Model file for the job. Use its own axes, mm. Face numbers are marked on the shaded views. A direction names the side the tool comes from. Give positions to 0.01 mm unless a question says otherwise; leave off trailing zeros. Write each loop counter-clockwise with the first axis right and the second up, starting at its lowest first coordinate (ties: lowest second). Pieces come first, ordered by that corner, then holes. Notation, with made-up numbers: (-25, -33) - (-17, -33) arc R26 ccw to (-17, 6) - close; hole circle Ø5 at (70, 41.5). An arc over 180 degrees is marked (long way). One line per item, written item: value. Start each with the question number.
(1) Drop flat-ended pins along their axis: P1, Ø2, axis at y = -4.5, z = -26.5, coming from the -X side; P2, Ø9, axis at x = 89, z = -82, coming from the +Y side; P3, Ø1.5, axis at y = -8, z = -61, coming from the +X side; P4, Ø1.5, axis at x = 46.5, z = -10.5, coming from the -Y side. Give the stop position or say it passes through.
(2) 3-axis set-ups, long thin cutter, end or side, ignore diameter. For the marked faces 1, 2 and 3: which of +Z, -Z, +X, -X, +Y, -Y reach the whole face in a straight line?
(3) Cut at B-B, the plane y = -10. List the corners of the cut face in (x, z) (3 decimals), and give its area (3 significant figures).
(4) Cut at A-A, the plane x = 32. List the corners of the cut face in (y, z) (3 decimals), and give its area (3 significant figures).
(5) Probe L1, parallel to Z at x = 35, y = 0.25; L2, parallel to X at y = -11.5, z = -58; L3, parallel to Y at x = 60.5, z = -10.5. List the from-to ranges inside material, lowest first.
(6) Cut at D-D, the plane x = 10. List the corners of the cut face in (y, z) (3 decimals).
(7) Cut at C-C, the plane z = -14.5. List the corners of the cut face in (x, y), and give its area (3 significant figures).
(8) Mould opens along X. For the marked faces 4, 5 and 6 say: pulls with the +X half, pulls with the -X half, needs draft (parallel to the pull), parting line crosses it, or undercut.
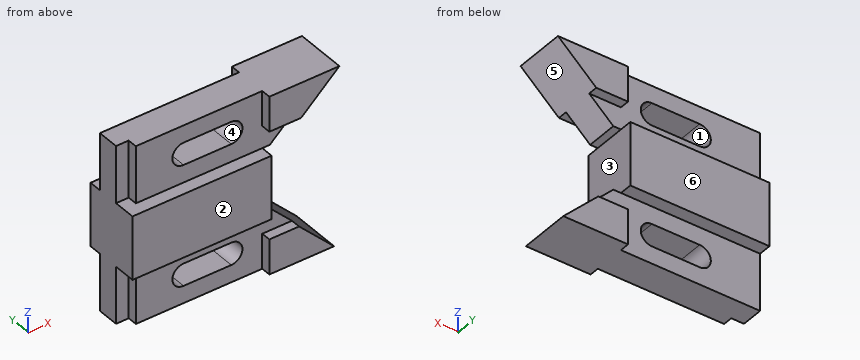
from build123d import *

# Parameters (mm, degrees)
F1_DEPTH = 14.224
F2_DEPTH = 7.874
F3_DEPTH = 12.7
F0_W     = 6.35
F0_H     = 28.575
F4_DEPTH = 7.874
F5_W     = 6.35
F5_H     = 28.575
F6_DEPTH = 4.826
F8_DEPTH = 22.099


with BuildPart() as f1:
    # F0 (on Front) → F1 (new body, symmetric)
    with BuildSketch(Plane.XZ):
        Polygon((6.35, -28.575), (0, -28.575), (0, -44.45), (0, -60.325), (6.35, -60.325), (69.596, -60.325), (69.596, -28.575), align=None)
    extrude(amount=F1_DEPTH, both=True)

    # F0 (on Front) → F2 (join, symmetric)
    with BuildSketch(Plane.XZ):
        Polygon((69.596, -60.325), (6.35, -60.325), (6.35, -88.9), (69.596, -88.9), (69.596, -71.374), (84.455, -71.374), (73.406, -60.325), align=None)
        Polygon((69.596, 0), (6.35, 0), (6.35, -28.575), (69.596, -28.575), (73.406, -28.575), (85.48624, -17.526), (69.596, -17.526), align=None)
    extrude(amount=F2_DEPTH, both=True)

    # F0 (on Front) → F3 (join, symmetric)
    with BuildSketch(Plane.XZ):
        Polygon((104.648, 0), (69.596, 0), (69.596, -17.526), (85.48624, -17.526), align=None)
        Polygon((69.596, -71.374), (69.596, -88.9), (101.981, -88.9), (84.455, -71.374), align=None)
    extrude(amount=F3_DEPTH, both=True)

    # F0 (on Front) → F4 (join, symmetric)
    with BuildSketch(Plane.XZ):
        with Locations((3.175, -14.2875)):
            Rectangle(F0_W, F0_H)
        Polygon((6.35, -28.575), (0, -28.575), (0, -44.45), (0, -60.325), (6.35, -60.325), (69.596, -60.325), (69.596, -28.575), align=None)
        with Locations((3.175, -74.6125)):
            Rectangle(F0_W, F0_H)
    extrude(amount=F4_DEPTH, both=True)

    # F5 (on face) → F6 (cut)
    with BuildSketch(Plane.XZ.offset(7.874)):
        with Locations((3.175, -14.2875)):
            Rectangle(F5_W, F5_H)
        with Locations((3.175, -74.6125)):
            Rectangle(F5_W, F5_H)
    extrude(amount=-F6_DEPTH, mode=Mode.SUBTRACT)

    # F7 (on face) → F8 (cut, through all)
    with BuildSketch(Plane.XZ.offset(7.874)):
        with BuildLine():
            Line((54.102, -8.636), (30.226, -8.636))
            ThreePointArc((30.226, -8.636), (24.638, -14.224), (30.226, -19.812))
            Line((30.226, -19.812), (54.102, -19.812))
            ThreePointArc((54.102, -19.812), (59.69, -14.224), (54.102, -8.636))
        make_face()
        with BuildLine():
            ThreePointArc((30.226, -69.088), (24.638, -74.676), (30.226, -80.264))
            Line((30.226, -80.264), (54.102, -80.264))
            ThreePointArc((54.102, -80.264), (59.69, -74.676), (54.102, -69.088))
            Line((54.102, -69.088), (30.226, -69.088))
        make_face()
    extrude(amount=-F8_DEPTH, mode=Mode.SUBTRACT)


solid = f1.part
Answers follow:
1. P1: stops at x = 6.35
1. P2: stops at y = 12.7
1. P3: stops at x = 74.82
1. P4: passes through
2. face 1: +Y, -Y
2. face 2: +Z, -Z, +X, -X, -Y
2. face 3: +X, +Y, -Y
3. outline: (0, -60.325) - (69.596, -60.325) - (69.596, -28.575) - (0, -28.575) - close; (69.596, -88.9) - (101.981, -88.9) - (84.455, -71.374) - (69.596, -71.374) - close; (69.596, -17.526) - (85.486, -17.526) - (104.648, 0) - (69.596, 0) - close
3. area: 3,070 mm²
4. outline: (-14.224, -60.325) - (-7.874, -60.325) - (-7.874, -69.088) - (7.874, -69.088) - (7.874, -60.325) - (14.224, -60.325) - (14.224, -28.575) - (7.874, -28.575) - (7.874, -19.812) - (-7.874, -19.812) - (-7.874, -28.575) - (-14.224, -28.575) - close; (-7.874, -88.9) - (7.874, -88.9) - (7.874, -80.264) - (-7.874, -80.264) - close; (-7.874, -8.636) - (7.874, -8.636) - (7.874, 0) - (-7.874, 0) - close
4. area: 1,450 mm²
5. L1: z = -88.9 to -80.26, -69.09 to -19.81, -8.64 to 0
5. L2: x = 0 to 69.6
5. L3: y = -7.87 to 7.87
6. outline: (-14.224, -60.325) - (-7.874, -60.325) - (-7.874, -88.9) - (7.874, -88.9) - (7.874, -60.325) - (14.224, -60.325) - (14.224, -28.575) - (7.874, -28.575) - (7.874, 0) - (-7.874, 0) - (-7.874, -28.575) - (-14.224, -28.575) - close
7. outline: (0, -3.05) - (6.35, -3.05) - (6.35, -7.87) - (24.64, -7.87) - (24.64, 7.87) - (0, 7.87) - close; (59.68, -7.87) - (69.6, -7.87) - (69.6, -12.7) - (88.79, -12.7) - (88.79, 12.7) - (69.6, 12.7) - (69.6, 7.87) - (59.68, 7.87) - close
7. area: 1,000 mm²
8. face 4: undercut
8. face 5: pulls with the +X half
8. face 6: needs draft
